The listing builds one solid part. Answer for the finished solid, in the listing's coordinates (mm). Coordinates: 2 decimals unless noted, no trailing zeros. Write each loop counter-clockwise with the first axis right and the second up, starting at its lowest first coordinate (ties: lowest second). Pieces come first, ordered by that corner, then holes. Notation, with made-up numbers: M 33,25.25 L 45,25.25 A8 cw 45,32.25 Z; hole C 79,83.5 d4. An arc over 180 degrees is marked long. Put each result on its own line as item: value. Start each with the question number.
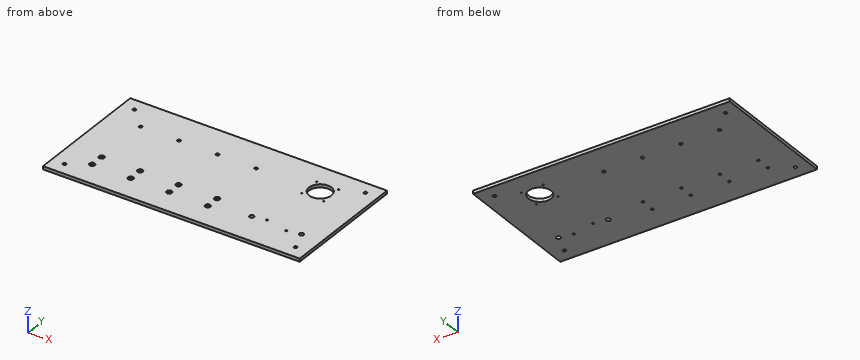
```python
from build123d import *

# Parameters (mm, degrees)
SKETCH_1_W          = 800
SKETCH_1_H          = 400
SKETCH_1_R          = 35
SKETCH_1_R_2        = 2
SKETCH_1_R_3        = 5
SKETCH_1_R_4        = 4
SKETCH_1_R_5        = 7
SKETCH_1_R_6        = 3
EXTRUDE_1_DEPTH     = 10
SKETCH_2_R          = 8.25
CUT_EXTRUDE_1_DEPTH = 4


with BuildPart() as part:
    # Эскиз1 → Бобышка-Вытянуть1 (new body)
    with BuildSketch(Plane.XY):
        with Locations((400, 200)):
            Rectangle(SKETCH_1_W, SKETCH_1_H)
        with Locations((660, 300)):
            Circle(SKETCH_1_R, mode=Mode.SUBTRACT)
        with Locations((626, 334)):
            Circle(SKETCH_1_R_2, mode=Mode.SUBTRACT)
        with Locations((694, 334)):
            Circle(SKETCH_1_R_2, mode=Mode.SUBTRACT)
        with Locations((694, 266)):
            Circle(SKETCH_1_R_2, mode=Mode.SUBTRACT)
        with Locations((626, 266)):
            Circle(SKETCH_1_R_2, mode=Mode.SUBTRACT)
        with Locations((100, 300)):
            Circle(SKETCH_1_R_3, mode=Mode.SUBTRACT)
        with Locations((220, 300)):
            Circle(SKETCH_1_R_3, mode=Mode.SUBTRACT)
        with Locations((340, 300)):
            Circle(SKETCH_1_R_3, mode=Mode.SUBTRACT)
        with Locations((460, 300)):
            Circle(SKETCH_1_R_3, mode=Mode.SUBTRACT)
        with Locations((100, 121.5)):
            Circle(SKETCH_1_R_4, mode=Mode.SUBTRACT)
        with Locations((220, 121.5)):
            Circle(SKETCH_1_R_4, mode=Mode.SUBTRACT)
        with Locations((340, 121.5)):
            Circle(SKETCH_1_R_4, mode=Mode.SUBTRACT)
        with Locations((460, 121.5)):
            Circle(SKETCH_1_R_4, mode=Mode.SUBTRACT)
        with Locations((460, 78.5)):
            Circle(SKETCH_1_R_4, mode=Mode.SUBTRACT)
        with Locations((340, 78.5)):
            Circle(SKETCH_1_R_4, mode=Mode.SUBTRACT)
        with Locations((220, 78.5)):
            Circle(SKETCH_1_R_4, mode=Mode.SUBTRACT)
        with Locations((100, 78.5)):
            Circle(SKETCH_1_R_4, mode=Mode.SUBTRACT)
        with Locations((582.5, 100)):
            Circle(SKETCH_1_R_5, mode=Mode.SUBTRACT)
        with Locations((737.5, 100)):
            Circle(SKETCH_1_R_5, mode=Mode.SUBTRACT)
        with Locations((625, 107.5)):
            Circle(SKETCH_1_R_6, mode=Mode.SUBTRACT)
        with Locations((695, 92.5)):
            Circle(SKETCH_1_R_6, mode=Mode.SUBTRACT)
        with Locations((40, 360)):
            Circle(SKETCH_1_R_3, mode=Mode.SUBTRACT)
        with Locations((760, 360)):
            Circle(SKETCH_1_R_3, mode=Mode.SUBTRACT)
        with Locations((760, 40)):
            Circle(SKETCH_1_R_3, mode=Mode.SUBTRACT)
        with Locations((40, 40)):
            Circle(SKETCH_1_R_3, mode=Mode.SUBTRACT)
    extrude(amount=EXTRUDE_1_DEPTH)

    # Эскиз2 → Вырез-Вытянуть1 (cut)
    with BuildSketch(Plane.XY.offset(10)):
        with Locations((100, 121.5)):
            Circle(SKETCH_2_R)
        with Locations((100, 78.5)):
            Circle(SKETCH_2_R)
        with Locations((220, 121.5)):
            Circle(SKETCH_2_R)
        with Locations((220, 78.5)):
            Circle(SKETCH_2_R)
        with Locations((340, 121.5)):
            Circle(SKETCH_2_R)
        with Locations((460, 121.5)):
            Circle(SKETCH_2_R)
        with Locations((460, 78.5)):
            Circle(SKETCH_2_R)
        with Locations((340, 78.5)):
            Circle(SKETCH_2_R)
    extrude(amount=-CUT_EXTRUDE_1_DEPTH, mode=Mode.SUBTRACT)


solid = part.part
```
1) A cutting plane is placed at B-B on x = 660. Write down the section's boundary in (y, z), then the cut area to 3 significant figures.
2) Given pin 1 Ø5 at (x, y) = (463.5, 79.5) entering from +Z, flat-ended and moving along its own axis, determine where the tip first touches the part or whether it passes through.
3) A cutting plane is placed at C-C on y = 323.5. Write down the section's boundary in (x, z), then the cut area to 3 significant figures.
4) A cutting plane is placed at A-A on z = 2.5. State how many separate pieces and enclosed holes the cut face has, then the cut area to 3 significant figures.
5) Straight lines are drawn through the part: probe 1 along X at (y, z) = (78.5, 1.4); probe 2 along Y at (x, z) = (340, 6.95); probe 3 along Y at (x, z) = (100, 3.8). For each, find the intervals that lie inside material, in ascending order.
Answers follow:
1. outline: M 0,0 L 265,0 L 265,10 L 0,10 Z; M 335,0 L 400,0 L 400,10 L 335,10 Z
1. area: 3,300 mm²
2. pin 1: stops at z = 6
3. outline: M 0,0 L 634.06,0 L 634.06,10 L 0,10 Z; M 685.94,0 L 800,0 L 800,10 L 685.94,10 Z
3. area: 7,480 mm²
4. separate pieces: 1
4. enclosed holes: 25
4. area: 315,000 mm²
5. probe 1: x = 0 to 96, 104 to 216, 224 to 336, 344 to 456, 464 to 800
5. probe 2: y = 0 to 70.25, 86.75 to 113.25, 129.75 to 295, 305 to 400
5. probe 3: y = 0 to 74.5, 82.5 to 117.5, 125.5 to 295, 305 to 400
